Design review of the part built by this model. Coordinates are the model's own, in mm. Face numbers are marked on the shaded views. A direction names the side the tool comes from. Coordinates: 2 decimals unless noted, no trailing zeros. Order: outer loops, then holes, each group sorted by start corner. A loop starts at its lowest first (then second) coordinate and runs counter-clockwise, first axis right, second up. Notation, with made-up numbers: M -15,15.25 L 32,15.25 A18 cw 32,43.25 Z; hole C 88.5,70.5 d4. An arc over 180 degrees is marked long. Use CSV: the item, a comma, the result in double quotes.
```python
from build123d import *

# Parameters (mm, degrees)
SKETCH1_W           = 71.12
SKETCH1_H           = 71.12
BOSS_EXTRUDE1_DEPTH = 4.7625
SKETCH2_R           = 3.4925
CUT_EXTRUDE1_DEPTH  = 51.514439582
SKETCH3_R           = 25.382
BOSS_EXTRUDE2_DEPTH = 83.5
SKETCH5_R           = 1.27
BOSS_EXTRUDE3_DEPTH = 10
FILLET1_R           = 2.5


with BuildPart() as part:
    # Sketch1 → Boss-Extrude1 (new body)
    with BuildSketch(Plane.XY):
        Rectangle(SKETCH1_W, SKETCH1_H)
    extrude(amount=BOSS_EXTRUDE1_DEPTH)

    # Sketch2 → Cut-Extrude1 (cut, through all)
    with BuildSketch(Plane.XY.offset(4.7625)):
        with Locations((-30.48, 30.48)):
            Circle(SKETCH2_R)
        with Locations((30.48, 30.48)):
            Circle(SKETCH2_R)
    cut_extrude1 = extrude(amount=-CUT_EXTRUDE1_DEPTH, mode=Mode.SUBTRACT)

    # Mirror1: Cut-Extrude1 across plane
    add(cut_extrude1.mirror(Plane.ZX), mode=Mode.SUBTRACT)

    # Sketch3 → Boss-Extrude2 (add)
    with BuildSketch(Plane.XY.offset(4.7625)):
        with Locations(Location((0, 0, 0), (0, 0, 180))):
            Circle(SKETCH3_R)
    extrude(amount=BOSS_EXTRUDE2_DEPTH)

    # Sketch4 → Cut-Revolve1 (revolve, cut)
    with BuildSketch(Plane(origin=(0, 0, 0), x_dir=(0, 0, -1), z_dir=(1, 0, 0)), mode=Mode.PRIVATE) as cut_revolve1_sk:
        Polygon((-4.7625, 25.382), (-88.2625, 1.245), (-88.2625, 25.382), align=None)
    revolve(cut_revolve1_sk.sketch.rotate(Axis((0, 0, 88.2625), (0, 0, -1)), 270), axis=Axis((0, 0, 88.2625), (0, 0, -1)), mode=Mode.SUBTRACT)

    # Sketch5 → Boss-Extrude3 (add)
    with BuildSketch(Plane.XY.offset(88.2625)):
        Circle(SKETCH5_R)
    extrude(amount=BOSS_EXTRUDE3_DEPTH)

    # Fillet1
    fillet1_edges = [part.edges().sort_by_distance(p)[0] for p in [
        (-35.56, 35.56, 2.38125),
        (35.56, 35.56, 2.38125),
        (35.56, -35.56, 2.38125),
        (-35.56, -35.56, 2.38125),
    ]]
    fillet(fillet1_edges, radius=FILLET1_R)


solid = part.part
```
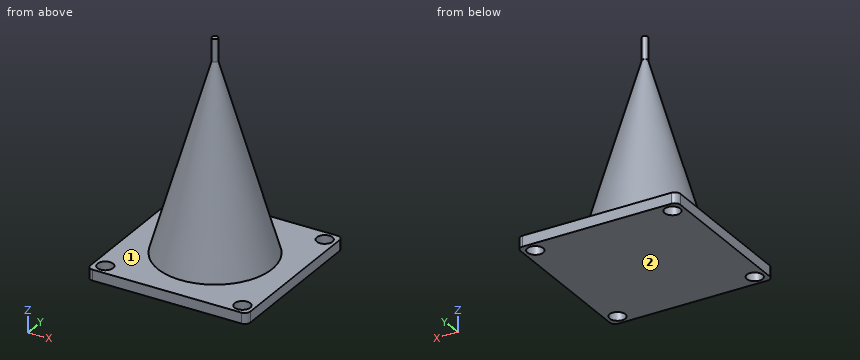
(1) Add section A-A on y = 30.48. State the section outline as (x, z) points.
The answers:
outline,"M -35.56,0 L -33.97,0 L -33.97,4.76 L -35.56,4.76 Z; M -26.99,0 L 26.99,0 L 26.99,4.76 L -26.99,4.76 Z; M 33.97,0 L 35.56,0 L 35.56,4.76 L 33.97,4.76 Z"
(2) Add section D-D on z = 13. State the section outline as (x, y) points.
The answers:
outline,"C 0,0 d46"
(3) For the marked faces 1 and 2, list the 3-axis set-ups (+Z, -Z, +X, -X, +Y, -Y) from which the entire face can be reached by the end or side of a thin tool; tool diameter is ignored.
The answers:
face 1,"+Z"
face 2,"-Z, +X, -X, +Y, -Y"
(4) Clearance check with flat-ended pins moving along their axes: P1, Ø9, axis at x = 30.48, y = 30.48, coming from the +Z side; P2, Ø5.5, axis at x = -30.48, y = 30.48, coming from the +Z side; P3, Ø4, axis at x = 10, z = 24.5, coming from the +Y side; P4, Ø1.5, axis at y = 6.5, z = 68, coming from the +X side. State where each tip first meets the part, or that it passes through.
The answers:
P1,"stops at z = 4.76"
P2,"passes through"
P3,"stops at y = 18.18"
P4,"stops at x = 4.23"
(5) Wall thickness on probe 1 along Y at (x, z) = (-30.48, 1.7); probe 2 along Z at (x, y) = (-17.5, 24); probe 3 along Y at (x, z) = (-30, 3): over which ranges is each line inside the solid? List them lowest first.
The answers:
probe 1,"y = -35.56 to -33.97, -26.99 to 26.99, 33.97 to 35.56"
probe 2,"z = 0 to 4.76"
probe 3,"y = -35.56 to -33.94, -27.02 to 27.02, 33.94 to 35.56"
